```python
from build123d import *

# Parameters (mm, degrees)
F1_DEPTH = 3


# Not quite as in the source:
# - ends of sketch curves that miss each other by under 0.0002 mm in the source are joined


with BuildPart() as f1:
    # F0 (on Top) → F1 (new body)
    with BuildSketch(Plane.XY):
        with BuildLine():
            ThreePointArc((32.9074971055, 11.248177677), (26.6878329895, 16.4993586176), (25.2500089531, 24.5113362153))
            ThreePointArc((25.2500089531, 24.5113362153), (-0.3819362324, 54.8706200704), (-26.0138819919, 24.5113361177))
            ThreePointArc((-26.0138819919, 24.5113361177), (-27.4517054543, 16.4993586176), (-33.6713695703, 11.248177677))
            ThreePointArc((-33.6713695703, 11.248177677), (-47.1473080368, -26.1293799296), (-8.0394240132, -33.1476541294))
            ThreePointArc((-8.0394240132, -33.1476541294), (-0.3819362324, -30.3868579581), (7.2755513239, -33.1476544003))
            ThreePointArc((7.2755513239, -33.1476544003), (46.383435572, -26.1293799296), (32.9074971055, 11.248177677))
        make_face()
    extrude(amount=-F1_DEPTH)


solid = f1.part
```
Here's how the part is built. I have some questions about the finished solid (model axes, mm). Give positions to 0.01 mm unless a question says otherwise; leave off trailing zeros. Write each loop counter-clockwise with the first axis right and the second up, starting at its lowest first coordinate (ties: lowest second). Pieces come first, ordered by that corner, then holes. Notation, with made-up numbers: M 43.5,74.25 L 58.5,74.25 A20 cw 58.5,86.25 Z; hole C -32.5,81 d7. An arc over 180 degrees is marked long. Put each result on its own line as item: value. Start each with the question number.
Item 1: If we section it at B-B, the plane y = -27: Write out the boundary of the cut face in (x, z), then the cut area to 3 significant figures.
Item 2: I need wall thicknesses on L1, parallel to X at y = -31.5, z = -1.45; L2, parallel to X at y = -34, z = -0.1; L3, parallel to X at y = -14, z = -0.45. Which ranges of each line are inside material? Lowest first, please. Write a range as from..to.
Item 3: If we section it at A-A, the plane z = -0.75: Write out the boundary of the cut face in (x, y), then the cut area to 3 significant figures.
Item 4: Will these pins go through, and if not, where does the flat tip stop? pin 1 (1.5 mm diameter, centred on y = -23, z = -2.5, fed in from -X); pin 2 (1.5 mm diameter, centred on x = -18, z = -2, fed in from +Y).
Item 5: Thinking about a two-plate mould opening in Y: for faces 1 (the cylindrical face through (-0.498, -30.387, -1.479)), 2 (the cylindrical face through (-27.394, 16.6, -1.479)), 3 (the cylindrical face through (26.746, 16.399, -1.479)), 4 (the flat face through (-1, -2, -3)), which applies, +Y half, -Y half, draft (parallel to the pull), parting line (faces both ways), or undercut?
Item 6: If we section it at C-C, the plane x = 14: Write out the boundary of the cut face in (y, z), then the cut area to 3 significant figures.
Values:
1. outline: M -46.62,-3 L 45.86,-3 L 45.86,0 L -46.62,0 Z
1. area: 277 mm²
2. L1: -43.03..-5.43, 4.67..42.27
2. L2: -40.14..-9.13, 8.36..39.37
2. L3: -50.62..49.85
3. outline: M -33.67,11.25 A26 ccw long -8.04,-33.15 A12 cw 7.28,-33.15 A26 ccw long 32.91,11.25 A12 cw 25.25,24.51 A26 ccw long -26.01,24.51 A12 cw Z
3. area: 6,380 mm²
4. pin 1: x = -48.98
4. pin 2: y = 48.66
5. face 1: -Y half
5. face 2: undercut
5. face 3: undercut
5. face 4: draft
6. outline: M -37.18,-3 L 50.53,-3 L 50.53,0 L -37.18,0 Z
6. area: 263 mm²
